For this review, use the dimensioned drawing (mm, ordinates from the lowest corner) and the shaded views. Round coordinates to 2 decimals unless told otherwise and drop trailing zeros. Write each loop counter-clockwise with the first axis right and the second up, starting at its lowest first coordinate (ties: lowest second). Pieces come first, ordered by that corner, then holes.
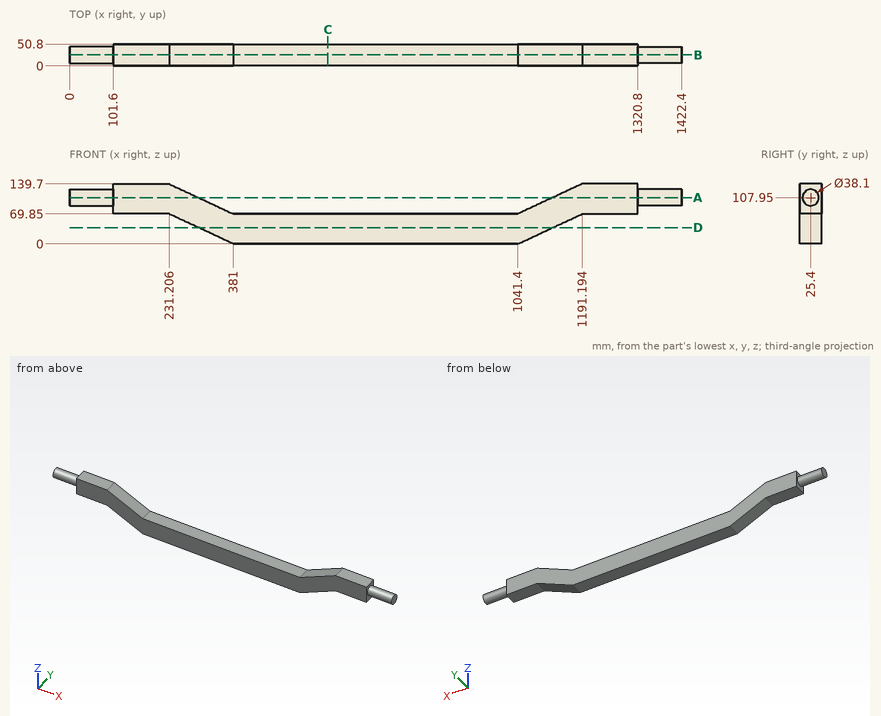
1) Add section B-B on y = 25.4. State the section outline as (x, z) points.
2) Add section A-A on z = 107.95. State the section outline as (x, y) points, and give its area (3 significant figures).
3) For line 1 along Z through (x, y) = (1035, 29); line 2 along Z through (x, y) = (178, 44); line 3 along X through (y, z) = (24.5, 130.5) (1 decimal), list the stretches that pass through material, from the lowest coordinate up.
4) Add section D-D on z = 38. State the section outline as (x, y) points.
5) For P1, Ø8, axis at y = 24, z = 54, coming from the -X side; P2, Ø12, axis at x = 264, y = 36.5, coming from the +Z side; P3, Ø15, axis at x = 1260.5, y = 20, coming from the -Z side, all flat-tipped, find the tip position at first contact; note any pin that passes through.
6) Add section C-C on x = 600.5. State the section outline as (y, z) points.
Computed:
1. outline: (0, 88.9) - (101.6, 88.9) - (101.6, 69.85) - (231.21, 69.85) - (381, 0) - (1041.4, 0) - (1191.19, 69.85) - (1320.8, 69.85) - (1320.8, 88.9) - (1422.4, 88.9) - (1422.4, 127) - (1320.8, 127) - (1320.8, 139.7) - (1191.19, 139.7) - (1041.4, 69.85) - (381, 69.85) - (231.21, 139.7) - (101.6, 139.7) - (101.6, 127) - (0, 127) - close
2. outline: (0, 6.35) - (101.6, 6.35) - (101.6, 0) - (299.29, 0) - (299.29, 50.8) - (101.6, 50.8) - (101.6, 44.45) - (0, 44.45) - close; (1123.11, 0) - (1320.8, 0) - (1320.8, 6.35) - (1422.4, 6.35) - (1422.4, 44.45) - (1320.8, 44.45) - (1320.8, 50.8) - (1123.11, 50.8) - close
2. area: 27,800 mm2
3. line 1: z = 0 to 69.85
3. line 2: z = 69.85 to 139.7
3. line 3: x = 101.6 to 250.9, 1171.5 to 1320.8
4. outline: (299.51, 0) - (1122.89, 0) - (1122.89, 50.8) - (299.51, 50.8) - close
5. P1: stops at x = 256.62
5. P2: stops at z = 127.21
5. P3: stops at z = 69.85
6. outline: (0, 0) - (50.8, 0) - (50.8, 69.85) - (0, 69.85) - close
